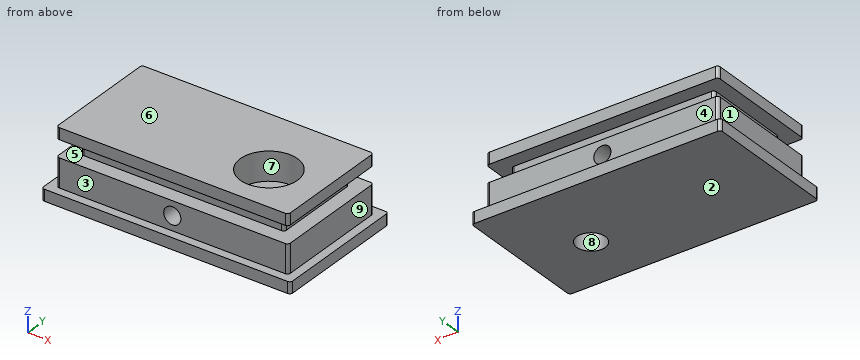
from build123d import *

# Parameters (mm, degrees)
F0_W      = 43.5
F0_H      = 23.5
F1_DEPTH  = 2
F2_W      = 40.5
F2_H      = 20.5
F3_DEPTH  = 5
F4_W      = 35.5
F4_H      = 15.5
F5_DEPTH  = 3
F6_W      = 40.5
F6_H      = 20.5
F7_DEPTH  = 2
F8_R      = 0.5
F9_R      = 2.5
F10_DEPTH = 12.001
F11_R     = 5
F12_DEPTH = 5
F13_R     = 1.5
F14_DEPTH = 25


with BuildPart() as f1:
    # F0 (on Top) → F1 (new body)
    with BuildSketch(Plane.XY):
        Rectangle(F0_W, F0_H)
    extrude(amount=F1_DEPTH)

    # F2 (on face) → F3 (join)
    with BuildSketch(Plane.XY.offset(2)):
        Rectangle(F2_W, F2_H)
    extrude(amount=F3_DEPTH)

    # F4 (on face) → F5 (join)
    with BuildSketch(Plane.XY.offset(7)):
        Rectangle(F4_W, F4_H)
    extrude(amount=F5_DEPTH)

    # F6 (on face) → F7 (join)
    with BuildSketch(Plane.XY.offset(10)):
        Rectangle(F6_W, F6_H)
    extrude(amount=F7_DEPTH)

    # F8
    f8_edges = [f1.edges().sort_by_distance(p)[0] for p in [
        (-20.25, 10.25, 4.5),
        (-17.75, 7.75, 8.5),
        (-20.25, 10.25, 11),
        (-20.25, -10.25, 4.5),
        (-17.75, -7.75, 8.5),
        (-20.25, -10.25, 11),
        (20.25, -10.25, 4.5),
        (17.75, -7.75, 8.5),
        (20.25, -10.25, 11),
        (20.25, 10.25, 4.5),
        (17.75, 7.75, 8.5),
        (20.25, 10.25, 11),
        (21.75, -11.75, 1),
        (21.75, 11.75, 1),
        (-21.75, -11.75, 1),
        (-21.75, 11.75, 1),
    ]]
    fillet(f8_edges, radius=F8_R)

    # F9 (on Top) → F10 (cut, through all)
    with BuildSketch(Plane.XY):
        with Locations((10.875, -2)):
            Circle(F9_R)
    extrude(amount=F10_DEPTH, mode=Mode.SUBTRACT)

    # F11 (on face) → F12 (cut, through all)
    with BuildSketch(Plane.XY.offset(12)):
        with Locations((10.875, -2)):
            Circle(F11_R)
    extrude(amount=-F12_DEPTH, mode=Mode.SUBTRACT)

    # F13 (on face) → F14 (cut)
    with BuildSketch(Plane.XZ.offset(10.25)):
        with Locations((0, 4.5)):
            Circle(F13_R)
    extrude(amount=-F14_DEPTH, mode=Mode.SUBTRACT)


solid = f1.part
Can you work these out from the model? Positions are in its coordinate system, mm. Face numbers are marked on the shaded views. A direction names the side the tool comes from. Round coordinates to 2 decimals unless told otherwise and drop trailing zeros. Order: outer loops, then holes, each group sorted by start corner. A loop starts at its lowest first (then second) coordinate and runs counter-clockwise, first axis right, second up. Notation, with made-up numbers: (2.25, 86) -> (61.25, 86) arc R32 ccw to (61.25, 121) -> close; hole circle Ø10 at (1, -28). An arc over 180 degrees is marked (long way). Write each question's results on one line, items separated by ' | '. Start each with the question number.
Item 1: If we section it at A-A, the plane y = -2: Write out the boundary of the cut face in (x, z) (3 decimals).
Item 2: Thinking about a two-plate mould opening in X: for the marked faces 6, 7, 8 and 9, which applies, +X half, -X half, draft (parallel to the pull), parting line (faces both ways), or undercut?
Item 3: If we section it at D-D, the plane y = -8.5: Write out the boundary of the cut face in (x, z).
Item 4: Which directions (+Z, -Z, +X, -X, +Y, -Y) give clear straight access to the entire face, cutting with the end or side of a thin tool? Please do the marked faces 1, 2, 3, 4 and 5.
Item 5: Will these pins go through, and if not, where does the flat tip stop? pin 1 (2.5 mm diameter, centred on y = 0.5, z = 9, fed in from +X); pin 2 (3 mm diameter, centred on x = 14, z = 6, fed in from +Y); pin 3 (5 mm diameter, centred on y = 5.5, z = 9.5, fed in from -X).
Item 6: If we section it at C-C, the plane z = 5: Write out the boundary of the cut face in (x, y) (3 decimals), then the cut area to 3 significant figures.
Item 7: Please list where these lines run through material, in increasing order: L1, parallel to Z at x = 0, y = -4.5; L2, parallel to Z at x = 5, y = -10; L3, parallel to X at y = -2, z = 4 (3 decimals).
Item 8: If we section it at B-B, the plane x = -19: Write out the boundary of the cut face in (y, z), then the cut area to 4 significant figures.
Results:
1) outline: (-21.75, 0) -> (8.375, 0) -> (8.375, 7) -> (5.875, 7) -> (5.875, 12) -> (-20.25, 12) -> (-20.25, 10) -> (-17.75, 10) -> (-17.75, 7) -> (-20.25, 7) -> (-20.25, 2) -> (-21.75, 2) -> close; (13.375, 0) -> (21.75, 0) -> (21.75, 2) -> (20.25, 2) -> (20.25, 7) -> (17.75, 7) -> (17.75, 10) -> (20.25, 10) -> (20.25, 12) -> (15.875, 12) -> (15.875, 7) -> (13.375, 7) -> close; hole circle Ø3 at (0, 4.5)
2) face 6: draft | face 7: undercut | face 8: undercut | face 9: +X half
3) outline: (-21.75, 0) -> (21.75, 0) -> (21.75, 2) -> (20.25, 2) -> (20.25, 7) -> (-20.25, 7) -> (-20.25, 2) -> (-21.75, 2) -> close; (-20.25, 10) -> (20.25, 10) -> (20.25, 12) -> (-20.25, 12) -> close; hole circle Ø3 at (0, 4.5)
4) face 1: +Z, -X, +Y, -Y | face 2: -Z, +X, -X, +Y, -Y | face 3: +Z, +X, -X, -Y | face 4: +Z, +X, -X, +Y | face 5: none
5) pin 1: stops at x = 20.25 | pin 2: stops at y = 10.25 | pin 3: stops at x = -20.25
6) outline: (-20.25, -9.75) arc R0.5 ccw to (-19.75, -10.25) -> (-1.414, -10.25) -> (-1.414, 10.25) -> (-19.75, 10.25) arc R0.5 ccw to (-20.25, 9.75) -> close; (1.414, -10.25) -> (19.75, -10.25) arc R0.5 ccw to (20.25, -9.75) -> (20.25, 9.75) arc R0.5 ccw to (19.75, 10.25) -> (1.414, 10.25) -> close; hole circle Ø5 at (10.875, -2) | area: 752 mm2
7) L1: z = 0 to 3, 6 to 12 | L2: z = 0 to 7, 10 to 12 | L3: x = -20.25 to -1.414, 1.414 to 8.375, 13.375 to 20.25
8) outline: (-11.75, 0) -> (11.75, 0) -> (11.75, 2) -> (10.25, 2) -> (10.25, 7) -> (-10.25, 7) -> (-10.25, 2) -> (-11.75, 2) -> close; (-10.25, 10) -> (10.25, 10) -> (10.25, 12) -> (-10.25, 12) -> close | area: 190.5 mm2
